from build123d import *

# Parameters (mm, degrees)
SKETCH005_W     = 16
SKETCH005_H     = 23.6
PAD001_DEPTH    = 1.6
SKETCH006_W     = 28.2
SKETCH006_H     = 23.6
PAD002_DEPTH    = 2
SKETCH007_W     = 1.9812
SKETCH007_H     = 1.27
POCKET002_DEPTH = 3.601
SKETCH008_R     = 4
SKETCH008_R_2   = 2.5
PAD003_DEPTH    = 8.6
SKETCH009_R     = 1.7
POCKET003_DEPTH = 2


with BuildPart() as part:
    # Sketch005 → Pad001 (new body)
    with BuildSketch(Plane.XY):
        with Locations((0, -33.4375)):
            Rectangle(SKETCH005_W, SKETCH005_H)
    extrude(amount=PAD001_DEPTH)

    # Sketch006 (on Face6 of Pad001) → Pad002 (join)
    with BuildSketch(Plane.XY.offset(1.6)):
        with Locations((0, -33.4375)):
            Rectangle(SKETCH006_W, SKETCH006_H)
    extrude(amount=PAD002_DEPTH)

    # Sketch007 (on Face7 of Pad002) → Pocket002 (cut, through all)
    with BuildSketch(Plane.XY.offset(3.6)):
        with Locations((-6.1781, -26.6025)):
            Rectangle(SKETCH007_W, SKETCH007_H)
        with Locations((6.1781, -26.6025)):
            Rectangle(SKETCH007_W, SKETCH007_H)
    extrude(amount=-POCKET002_DEPTH, mode=Mode.SUBTRACT)

    # Sketch008 (on Face7 of Pocket002) → Pad003 (join)
    with BuildSketch(Plane.XY.offset(3.6)):
        with Locations((-6.1781, -26.6025)):
            Circle(SKETCH008_R)
        with Locations((-6.1781, -26.6025)):
            Circle(SKETCH008_R_2, mode=Mode.SUBTRACT)
        with Locations((6.1781, -26.6025)):
            Circle(SKETCH008_R)
        with Locations((6.1781, -26.6025)):
            Circle(SKETCH008_R_2, mode=Mode.SUBTRACT)
    extrude(amount=PAD003_DEPTH)

    # Sketch009 (on Face7 of Pad003) → Pocket003 (cut)
    with BuildSketch(Plane.XY.offset(3.6)):
        with Locations((-11.1, -42.2375)):
            Circle(SKETCH009_R)
        with Locations((11.1, -42.2375)):
            Circle(SKETCH009_R)
        with Locations((-11.1, -33.2375)):
            Circle(SKETCH009_R)
        with Locations((11.1, -33.2375)):
            Circle(SKETCH009_R)
    extrude(amount=-POCKET003_DEPTH, mode=Mode.SUBTRACT)


with BuildPart() as part_1:
    # Body001 placement: moved
    add(part.part.moved(Location((0, 0, 2.4))))


solid = part_1.part
Design review of the part built by this model. Coordinates are the model's own, in mm. A direction names the side the tool comes from. Coordinates: 2 decimals unless noted, no trailing zeros. Loops run counter-clockwise (first coordinate to the right, second up) from the corner with the lowest first, then second, coordinate; pieces in that order, holes last.
Item 1: Wall thickness on L1, parallel to Y at x = 11.1, z = 4.95; L2, parallel to X at y = -28.5, z = 11.5; L3, parallel to Z at x = 3.5, y = -41.75: over which ranges is each line inside the solid? List them lowest first.
Completed:
L1: y = -45.24 to -43.94, -40.54 to -34.94, -31.54 to -21.64
L2: x = -9.7 to -7.81, -4.55 to -2.66, 2.66 to 4.55, 7.81 to 9.7
L3: z = 2.4 to 6
Item 2: Add section B-B (x = 6.5). Write out the cut boundary in (y, z).
Completed:
outline: (-45.24, 2.4) - (-27.24, 2.4) - (-27.24, 6) - (-29.08, 6) - (-29.08, 14.6) - (-30.59, 14.6) - (-30.59, 6) - (-45.24, 6) - close; (-25.97, 2.4) - (-21.64, 2.4) - (-21.64, 6) - (-22.62, 6) - (-22.62, 14.6) - (-24.12, 14.6) - (-24.12, 6) - (-25.97, 6) - close
Item 3: Draft analysis for pull direction Y (two halves, no side actions). For faces 5 (the cylindrical face through (-6.699, -22.637, 10.24)), 6 (the cylindrical face through (12.01, -31.8, 5.01)), 7 (the flat face through (6, -28, 6)), 8 (the flat face through (14.1, -34, 5)), state which applies: pulls with the +Y half, pulls with the -Y half, needs draft (parallel to the pull), parting line crosses it, or undercut.
Completed:
face 5: parting line crosses it
face 6: undercut
face 7: undercut
face 8: needs draft
Item 4: Add section D-D (z = 5). Write out the cut boundary in (x, y), and give its area (3 significant figures).
Completed:
outline: (-14.1, -45.24) - (14.1, -45.24) - (14.1, -21.64) - (-14.1, -21.64) - close; hole circle Ø3.4 at (-11.1, -42.24); hole circle Ø3.4 at (-11.1, -33.24); hole (-7.17, -27.24) - (-5.19, -27.24) - (-5.19, -25.97) - (-7.17, -25.97) - close; hole (5.19, -27.24) - (7.17, -27.24) - (7.17, -25.97) - (5.19, -25.97) - close; hole circle Ø3.4 at (11.1, -42.24); hole circle Ø3.4 at (11.1, -33.24)
area: 624 mm2
Item 5: Add section A-A (x = 11.1). Write out the cut boundary in (y, z).
Completed:
outline: (-45.24, 4) - (-43.94, 4) - (-43.94, 6) - (-45.24, 6) - close; (-40.54, 4) - (-34.94, 4) - (-34.94, 6) - (-40.54, 6) - close; (-31.54, 4) - (-21.64, 4) - (-21.64, 6) - (-31.54, 6) - close
Item 6: Clearance check with flat-ended pins moving along their axes: pin 1 (2.5 mm diameter, centred on x = 11.1, y = -42.24, fed in from +Z); pin 2 (5 mm diameter, centred on x = -1, z = 10, fed in from +Y); pin 3 (1.8 mm diameter, centred on y = -32.5, z = 3, fed in from +X); pin 4 (4.5 mm diameter, centred on x = -11.1, y = -42.24, fed in from +Z). State where each tip first meets the part, or that it passes through.
Completed:
pin 1: passes through
pin 2: stops at y = -23.63
pin 3: stops at x = 8
pin 4: stops at z = 6
Item 7: For faces 1 (the flat face through (11, -31, 4)), 2 (the flat face through (-8, -34, 3)), 3 (the flat face through (0, -33, 2.4)), 4 (the flat face through (-6, -25.967, 4)), list the 3-axis set-ups (+Z, -Z, +X, -X, +Y, -Y) from which the entire face can be reached by the end or side of a thin tool; tool diameter is ignored.
Completed:
face 1: -Z, +X, +Y, -Y
face 2: -Z, -X, +Y, -Y
face 3: -Z, +X, -X, +Y, -Y
face 4: +Z, -Z
Item 8: Add section C-C (y = -35.25). Write out the cut boundary in (x, z), and give its area (3 significant figures).
Completed:
outline: (-14.1, 4) - (-8, 4) - (-8, 2.4) - (8, 2.4) - (8, 4) - (14.1, 4) - (14.1, 6) - (-14.1, 6) - close
area: 82.0 mm2
